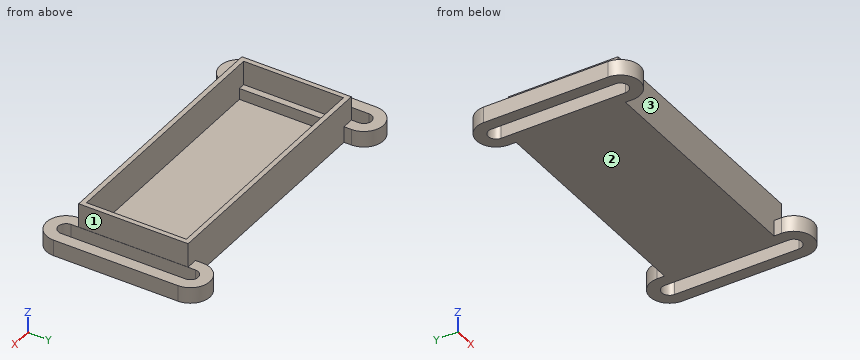
```python
from build123d import *

# Parameters (mm, degrees)
BOSS_EXTRUDE1_DEPTH = 10
SKETCH2_W           = 63.9
SKETCH2_H           = 27.3
BOSS_EXTRUDE2_DEPTH = 1.2
BOSS_EXTRUDE3_DEPTH = 4


with BuildPart() as part:
    # 3DSketch1 → Boss-Extrude1 (new body)
    with BuildSketch(Plane(origin=(-40.430283892, 18.807335645, 0), x_dir=(0.9232075579857172, -0.3843017107404659, 0), z_dir=(0, 0, 1))):
        Polygon((-1.569011122, 0.646687017), (57.423951833, 25.203566333), (67.915388536, 0), (8.922425581, -24.556879316), align=None)
        Polygon((0, 0), (56.777264816, 23.634555211), (66.346377414, 0.646687017), (9.569112597, -22.987868194), align=None, mode=Mode.SUBTRACT)
    extrude(amount=BOSS_EXTRUDE1_DEPTH)

    # Sketch2 → Boss-Extrude2 (add)
    with BuildSketch(Plane(origin=(0, 0, 0), x_dir=(-1, 0, 0), z_dir=(0, 0, -1))):
        with Locations((9.680283892, 6.357335645)):
            Rectangle(SKETCH2_W, SKETCH2_H)
    extrude(amount=-BOSS_EXTRUDE2_DEPTH)

    # Sketch4 → Boss-Extrude3 (add)
    with BuildSketch(Plane(origin=(0, 0, 0), x_dir=(-1, 0, 0), z_dir=(0, 0, -1))):
        with BuildLine():
            Line((48.507458783, 21.857335645), (48.507458783, -9.142664355))
            ThreePointArc((48.507458783, -9.142664355), (43.630283892, -14.019839246), (38.753109001, -9.142664355))
            Line((38.753109001, -9.142664355), (38.753109001, 21.857335645))
            ThreePointArc((38.753109001, 21.857335645), (43.630283892, 26.734510536), (48.507458783, 21.857335645))
        make_face()
        with BuildLine():
            Line((45.58467524, 21.857335645), (45.58467524, -9.142664355))
            ThreePointArc((45.58467524, -9.142664355), (43.630283892, -11.097055703), (41.675892544, -9.142664355))
            Line((41.675892544, -9.142664355), (41.675892544, 21.857335645))
            ThreePointArc((41.675892544, 21.857335645), (43.630283892, 23.811726993), (45.58467524, 21.857335645))
        make_face(mode=Mode.SUBTRACT)
        with BuildLine():
            Line((-29.146890999, 21.857335645), (-29.146890999, -9.142664355))
            ThreePointArc((-29.146890999, -9.142664355), (-24.269716108, -14.019839246), (-19.392541217, -9.142664355))
            Line((-19.392541217, -9.142664355), (-19.392541217, 21.857335645))
            ThreePointArc((-19.392541217, 21.857335645), (-24.269716108, 26.734510536), (-29.146890999, 21.857335645))
        make_face()
        with BuildLine():
            Line((-26.224107456, 21.857335645), (-26.224107456, -9.142664355))
            ThreePointArc((-26.224107456, -9.142664355), (-24.269716108, -11.097055703), (-22.31532476, -9.142664355))
            Line((-22.31532476, -9.142664355), (-22.31532476, 21.857335645))
            ThreePointArc((-22.31532476, 21.857335645), (-24.269716108, 23.811726993), (-26.224107456, 21.857335645))
        make_face(mode=Mode.SUBTRACT)
    extrude(amount=-BOSS_EXTRUDE3_DEPTH)


solid = part.part
```
The model under review builds one solid part; all positions refer to its coordinate system, in mm. Face numbers are marked on the shaded views. Round coordinates to 2 decimals unless told otherwise and drop trailing zeros. Order: outer loops, then holes, each group sorted by start corner. A loop starts at its lowest first (then second) coordinate and runs counter-clockwise, first axis right, second up. Notation, with made-up numbers: (5, -34.5) - (14, -34.5) arc R12 ccw to (14, -16.5) - close; hole circle Ø8 at (-32.75, 38.25). An arc over 180 degrees is marked (long way). Answer in a Markdown table with one row per item.
(1) Take a section at D-D on z = 3.25. Write out the cut boundary in (x, y), plus the area to 3 significant figures.
Result set:
| item | result |
|---|---|
| outline | (-48.51, -9.14) arc R4.88 ccw to (-38.75, -9.14) - (-38.75, -7.29) - (19.39, -7.29) - (19.39, -9.14) arc R4.88 ccw to (29.15, -9.14) - (29.15, 21.86) arc R4.88 ccw to (19.39, 21.86) - (19.39, 20.01) - (-38.75, 20.01) - (-38.75, 21.86) arc R4.88 ccw to (-48.51, 21.86) - close; hole (-45.58, -9.14) arc R1.95 ccw to (-41.68, -9.14) - (-41.68, 21.86) arc R1.95 ccw to (-45.58, 21.86) - close; hole (-38.75, -6.09) - (19.39, -6.09) - (19.39, 18.81) - (-38.75, 18.81) - close; hole (22.32, -9.14) arc R1.95 ccw to (26.22, -9.14) - (26.22, 21.86) arc R1.95 ccw to (22.32, 21.86) - close |
| area | 627 mm2 |
(2) Take a section at B-B on z = 8.25. Write out the cut boundary in (x, y).
Result set:
| item | result |
|---|---|
| outline | (-41.63, -7.29) - (22.27, -7.29) - (22.27, 20.01) - (-41.63, 20.01) - close; hole (-40.43, -6.09) - (21.07, -6.09) - (21.07, 18.81) - (-40.43, 18.81) - close |
(3) Clearance check with flat-ended pins moving along their axes: P1, Ø3, axis at y = 4.5, z = 7, coming from the +X side; P2, Ø3, axis at x = -21, z = 4.5, coming from the -Y side; P3, Ø12, axis at x = -7.5, y = 5, coming from the -Z side; P4, Ø1.8, axis at x = 20, y = 10, coming from the +Z side. State where each tip first meets the part, or that it passes through.
Result set:
| item | result |
|---|---|
| P1 | stops at x = 22.27 |
| P2 | stops at y = -7.29 |
| P3 | stops at z = 0 |
| P4 | stops at z = 4 |
(4) Take a section at A-A on y = 7. Write out the cut boundary in (x, z).
Result set:
| item | result |
|---|---|
| outline | (-48.51, 0) - (-45.58, 0) - (-45.58, 4) - (-48.51, 4) - close; (-41.68, 0) - (22.32, 0) - (22.32, 4) - (22.27, 4) - (22.27, 10) - (21.07, 10) - (21.07, 4) - (19.39, 4) - (19.39, 1.2) - (-38.75, 1.2) - (-38.75, 4) - (-40.43, 4) - (-40.43, 10) - (-41.63, 10) - (-41.63, 4) - (-41.68, 4) - close; (26.22, 0) - (29.15, 0) - (29.15, 4) - (26.22, 4) - close |
(5) Take a section at C-C on x = -43. Write out the cut boundary in (y, z), plus the area to 3 significant figures.
Result set:
| item | result |
|---|---|
| outline | (-13.98, 0) - (-10.99, 0) - (-10.99, 4) - (-13.98, 4) - close; (23.71, 0) - (26.69, 0) - (26.69, 4) - (23.71, 4) - close |
| area | 23.9 mm2 |
(6) For line 1 (X direction, y = 7.5, z = 3); line 2 (X direction, y = 17, z = 0.5); line 3 (Y direction, x = -14.5, z = 1.5), list the stretches that pass through material, from the lowest coordinate up. Write a range as from..to.
Result set:
| item | result |
|---|---|
| line 1 | x = -48.51..-45.58, -41.68..-38.75, 19.39..22.32, 26.22..29.15 |
| line 2 | x = -48.51..-45.58, -41.68..22.32, 26.22..29.15 |
| line 3 | y = -7.29..-6.09, 18.81..20.01 |
(7) Mouldability with a two-part tool opening along X and no side actions: class the marked faces 1, 2 and 3 as released by +X, released by -X, zero draft, split by the parting line, or undercut.
Result set:
| item | result |
|---|---|
| face 1 | released by +X |
| face 2 | zero draft |
| face 3 | undercut |
